Build history of the part. All positions in model axes, mm. A direction names the side the tool comes from. Give positions to 0.01 mm unless a question says otherwise; leave off trailing zeros. Order: outer loops, then holes, each group sorted by start corner. A loop starts at its lowest first (then second) coordinate and runs counter-clockwise, first axis right, second up. Notation, with made-up numbers: (31.5, 39.5) - (80.5, 39.5) arc R12 ccw to (80.5, 52.5) - close; hole circle Ø11 at (66, 88.25). An arc over 180 degrees is marked (long way). Write each question's results on one line, items separated by ' | '. Start each with the question number.
1) Drill centre lines: line 1 along X through (y, z) = (4.75, 6.5); line 2 along X through (y, z) = (1.5, 4.25); line 3 along Z through (x, y) = (10.25, 1.4). Where is each one in solid material? Low to high. Write a range as from..to.
2) Cut at D-D on z = -3.5. List the corners of the cut face in (x, y).
3) Cut at C-C on y = 8.75. List the corners of the cut face in (x, z), plus the area to 3 significant figures.
4) Drop flat-ended pins along their axis: pin 1 Ø5.5 at (x, z) = (-12, -2) entering from +Y; pin 2 Ø1 at (y, z) = (5, 2) entering from +X; pin 3 Ø3.5 at (y, z) = (6.5, 0) entering from -X; pin 4 Ø1 at (x, y) = (4, 5) entering from -Z. Give the stop position or say it passes through.
5) Two-plate mould, pull along X, no slides. Class faces 6 (the face through (6.717, 0.697, 0.105)), 7 (the face through (-9.076, 3.046, 4.784)), 8 (the face through (0, 12, 0)): +X half, -X half, draft (parallel to the pull), parting line (faces both ways), or undercut.
6) Tool access for faces 1 (the face through (6, 3, 0)), 2 (the face through (-12, 2, 0)), 3 (the face through (-8, 7, 5)), 4 (the face through (8, 7, -5)), 5 (the face through (7.72, 5.36, 1.83)): list every direction of +Z, -Z, +X, -X, +Y, -Y with a clear straight run to the whole face (end or side of a thin tool).
7) Cut at A-A on z = 0. List the corners of the cut face in (x, y), plus the area to 3 significant figures.
8) Cut at B-B on x = -9.25. List the corners of the cut face in (y, z).
from build123d import *

# Parameters (mm, degrees)
SALIENTE_EXTRUIR1_DEPTH = 7.5
REDONDEO1_R             = 2
CORTAR_EXTRUIR2_DEPTH   = 10
CROQUIS4_R              = 1.5
CORTAR_EXTRUIR3_DEPTH   = 11


with BuildPart() as part:
    # Croquis1 → Saliente-Extruir1 (new body, symmetric)
    with BuildSketch(Plane.XY):
        with BuildLine():
            Line((14.5, 0), (7.414213562, 0))
            Line((7.414213562, 0), (6, 1.414213562))
            Line((6, 1.414213562), (6, 5))
            ThreePointArc((6, 5), (5.286764074, 7.837274331), (3.31662479, 10))
            Line((3.31662479, 10), (-3.31662479, 10))
            ThreePointArc((-3.31662479, 10), (-5.286764074, 7.837274331), (-6, 5))
            Line((-6, 5), (-6, 1.414213562))
            Line((-6, 1.414213562), (-7.414213562, 0))
            Line((-7.414213562, 0), (-14.5, 0))
            Line((-14.5, 0), (-14.5, 2))
            Line((-14.5, 2), (-10.121320344, 2))
            Line((-10.121320344, 2), (-8, 4.121320344))
            Line((-8, 4.121320344), (-8, 12))
            Line((-8, 12), (8, 12))
            Line((8, 12), (8, 4.121320344))
            Line((8, 4.121320344), (10.121320344, 2))
            Line((10.121320344, 2), (14.5, 2))
            Line((14.5, 2), (14.5, 0))
        make_face()
    extrude(amount=SALIENTE_EXTRUIR1_DEPTH, both=True)

    # Redondeo1
    redondeo1_edges = [part.edges().sort_by_distance(p)[0] for p in [
        (-8, 12, 0),
        (8, 12, 0),
    ]]
    fillet(redondeo1_edges, radius=REDONDEO1_R)

    # Croquis3 → Cortar-Extruir2 (cut)
    with BuildSketch(Plane(origin=(0, 12, 0), x_dir=(1, 0, 0), z_dir=(0, 1, 0))):
        Polygon((-10.15, -3.233161507), (-7.35, -1.616580754), (-7.35, 1.616580754), (-10.15, 3.233161507), (-12.95, 1.616580754), (-12.95, -1.616580754), align=None)
        Polygon((12.95, -1.616580754), (10.15, -3.233161507), (7.35, -1.616580754), (7.35, 1.616580754), (10.15, 3.233161507), (12.95, 1.616580754), align=None)
    extrude(amount=-CORTAR_EXTRUIR2_DEPTH, mode=Mode.SUBTRACT)

    # Croquis4 → Cortar-Extruir3 (cut)
    with BuildSketch(Plane.XZ):
        with Locations((-10.25, 0)):
            Circle(CROQUIS4_R)
        with Locations((10.25, 0)):
            Circle(CROQUIS4_R)
    extrude(amount=-CORTAR_EXTRUIR3_DEPTH, mode=Mode.SUBTRACT)


solid = part.part
Results:
1) line 1: -8..-6, 6..8 | line 2: -14.5..-6, 6..14.5 | line 3: -7.5..-1.5, 1.5..7.5
2) outline: (-14.5, 0) - (-7.41, 0) - (-6, 1.41) - (-6, 5) arc R6 cw to (-3.32, 10) - (3.32, 10) arc R6 cw to (6, 5) - (6, 1.41) - (7.41, 0) - (14.5, 0) - (14.5, 2) - (10.12, 2) - (8, 4.12) - (8, 10) arc R2 ccw to (6, 12) - (-6, 12) arc R2 ccw to (-8, 10) - (-8, 4.12) - (-10.12, 2) - (-14.5, 2) - close
3) outline: (-8, -7.5) - (-4.68, -7.5) - (-4.68, 7.5) - (-8, 7.5) - (-8, 1.99) - (-7.35, 1.62) - (-7.35, -1.62) - (-8, -1.99) - close; (4.68, -7.5) - (8, -7.5) - (8, -1.99) - (7.35, -1.62) - (7.35, 1.62) - (8, 1.99) - (8, 7.5) - (4.68, 7.5) - close | area: 94.8 mm^2
4) pin 1: y = 2.76 | pin 2: x = 8 | pin 3: x = -7.58 | pin 4: through
5) face 6: undercut | face 7: -X half | face 8: draft
6) face 1: +Z, -Z, -Y | face 2: -X, +Y | face 3: +Z, -Z, -X, +Y | face 4: +Z, -Z, +X, +Y | face 5: +X, +Y
7) outline: (-14.5, 0) - (-11.75, 0) - (-11.75, 2) - (-14.5, 2) - close; (-8.75, 0) - (-7.41, 0) - (-6, 1.41) - (-6, 5) arc R6 cw to (-3.32, 10) - (3.32, 10) arc R6 cw to (6, 5) - (6, 1.41) - (7.41, 0) - (8.75, 0) - (8.75, 2) - (7.35, 2) - (7.35, 11.48) arc R2 ccw to (6, 12) - (-6, 12) arc R2 ccw to (-7.35, 11.48) - (-7.35, 2) - (-8.75, 2) - close; (11.75, 0) - (14.5, 0) - (14.5, 2) - (11.75, 2) - close | area: 78.5 mm^2
8) outline: (0, -7.5) - (2.87, -7.5) - (2.87, -2.71) - (2, -2.71) - (2, -1.12) - (0, -1.12) - close; (0, 1.12) - (2, 1.12) - (2, 2.71) - (2.87, 2.71) - (2.87, 7.5) - (0, 7.5) - close
